For this review, use the dimensioned drawing (mm, ordinates from the lowest corner) and the shaded views. A direction names the side the tool comes from. Coordinates: 2 decimals unless noted, no trailing zeros. Write each loop counter-clockwise with the first axis right and the second up, starting at its lowest first coordinate (ties: lowest second). Pieces come first, ordered by that corner, then holes.
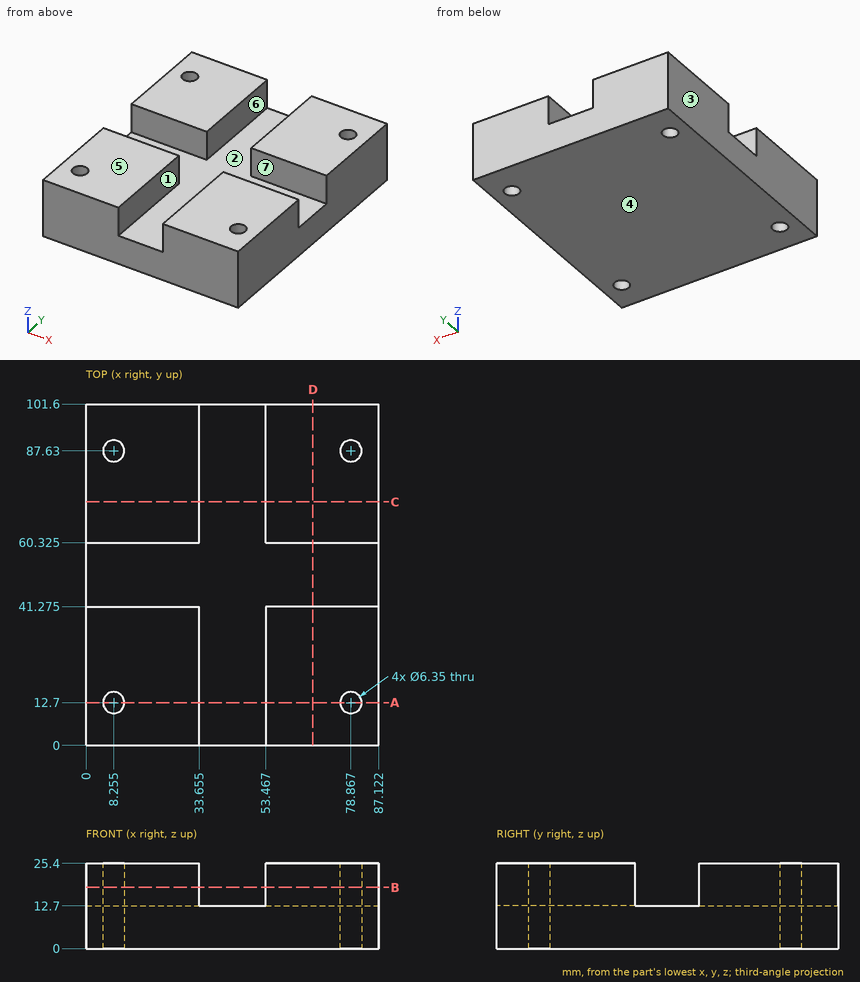
(1) Consider section B-B (z = 18.25). Give the boundary of the cut face in (x, y) (3 decimals), plus the area to 3 significant figures.
(2) For the marked faces 5, 6 and 7, list the 3-axis set-ups (+Z, -Z, +X, -X, +Y, -Y) from which the entire face can be reached by the end or side of a thin tool; tool diameter is ignored.
(3) Wall thickness on line 1 (X direction, y = 35, z = 18.75) (3 decimals); line 2 (X direction, y = 89, z = 14.5) (3 decimals); line 3 (Y direction, x = 7, z = 21.75) (3 decimals): over which ranges is each line inside the solid? List them lowest first.
(4) Consider section A-A (y = 12.7). Give the boundary of the cut face in (x, z) (3 decimals), plus the area to 3 significant figures.
(5) Consider section C-C (y = 72.5). Give the boundary of the cut face in (x, z) (3 decimals).
(6) Mouldability with a two-part tool opening along X and no side actions: class the marked faces 1, 2, 3 and 4 as +X half, -X half, draft (parallel to the pull), parting line (faces both ways), or undercut.
(7) Consider section D-D (x = 67.5). Give the boundary of the cut face in (y, z) (3 decimals), plus the area to 3 significant figures.
Results:
1. outline: (0, 0) - (33.655, 0) - (33.655, 41.275) - (0, 41.275) - close; (0, 60.325) - (33.655, 60.325) - (33.655, 101.6) - (0, 101.6) - close; (53.467, 0) - (87.122, 0) - (87.122, 41.275) - (53.467, 41.275) - close; (53.467, 60.325) - (87.122, 60.325) - (87.122, 101.6) - (53.467, 101.6) - close; hole circle Ø6.35 at (8.255, 12.7); hole circle Ø6.35 at (8.255, 87.63); hole circle Ø6.35 at (78.867, 12.7); hole circle Ø6.35 at (78.867, 87.63)
1. area: 5,430 mm2
2. face 5: +Z, +X, -X, +Y, -Y
2. face 6: +Z, +Y, -Y
2. face 7: +Z, +X, -X
3. line 1: x = 0 to 33.655, 53.467 to 87.122
3. line 2: x = 0 to 5.391, 11.119 to 33.655, 53.467 to 76.003, 81.731 to 87.122
3. line 3: y = 0 to 9.784, 15.616 to 41.275, 60.325 to 84.714, 90.546 to 101.6
4. outline: (0, 0) - (5.08, 0) - (5.08, 25.4) - (0, 25.4) - close; (11.43, 0) - (75.692, 0) - (75.692, 25.4) - (53.467, 25.4) - (53.467, 12.7) - (33.655, 12.7) - (33.655, 25.4) - (11.43, 25.4) - close; (82.042, 0) - (87.122, 0) - (87.122, 25.4) - (82.042, 25.4) - close
4. area: 1,640 mm2
5. outline: (0, 0) - (87.122, 0) - (87.122, 25.4) - (53.467, 25.4) - (53.467, 12.7) - (33.655, 12.7) - (33.655, 25.4) - (0, 25.4) - close
6. face 1: undercut
6. face 2: undercut
6. face 3: -X half
6. face 4: draft
7. outline: (0, 0) - (101.6, 0) - (101.6, 25.4) - (60.325, 25.4) - (60.325, 12.7) - (41.275, 12.7) - (41.275, 25.4) - (0, 25.4) - close
7. area: 2,340 mm2
